Check sheet for the modelled part. Datum: model origin and axes. Units: mm. A direction names the side the tool comes from. Coordinates: 2 decimals unless noted, no trailing zeros. Loops run counter-clockwise (first coordinate to the right, second up) from the corner with the lowest first, then second, coordinate; pieces in that order, holes last. Notation, with made-up numbers: (13.25, -2.75) -> (17.25, -2.75) arc R20 cw to (17.25, 2.25) -> close; hole circle Ø3 at (9, 38). An arc over 180 degrees is marked (long way). Use one line per item in the form item = value.
from build123d import *

# Parameters (mm, degrees)
F1_DEPTH = 26
F2_SIZE  = 0.8


with BuildPart() as f1:
    # F0 (on Front) → F1 (new body)
    with BuildSketch(Plane.XZ):
        Polygon((-14.5, 0), (0, 0), (0, 2), (-13, 2), (-13, 12), (-10, 12), (-10, 13.5), (-14.5, 13.5), align=None)
    extrude(amount=-F1_DEPTH)

    # F2
    f2_edges = [f1.edges().sort_by_distance(p)[0] for p in [
        (-10, 13, 12),
    ]]
    chamfer(f2_edges, length=F2_SIZE)

    # F3: F1 across plane


with BuildPart() as f1_1:
    add(f1.part)
    add(f1.part.mirror(Plane.YZ))


solid = f1_1.part
(1) Scan lines: line 1 along X through (y, z) = (6, 13); line 2 along X through (y, z) = (12.5, 8.75); line 3 along Z through (x, y) = (-11.25, 14.5). Record each from-to range of solid material in increasing order.
Established:
line_1 = -14.5 to -10, 10 to 14.5
line_2 = -14.5 to -13, 13 to 14.5
line_3 = 0 to 2, 12 to 13.5
(2) Mould release check, pull along X, two halves, no side actions. Record for faces 3 (the flat face through (12, 13, 13.5)), 4 (the flat face through (-13, 13, 7)), 5 (the flat face through (14.5, 13, 7)): +X half, -X half, draft (parallel to the pull), parting line (faces both ways), or undercut.
Established:
face_3 = draft
face_4 = undercut
face_5 = +X half
(3) Section check C-C, the plane x = -12.5. Record the boundary of the cut face in (y, z), plus the area to 3 significant figures.
Established:
outline = (0, 0) -> (26, 0) -> (26, 2) -> (0, 2) -> close; (0, 12) -> (26, 12) -> (26, 13.5) -> (0, 13.5) -> close
area = 91.0 mm²
(4) Section check D-D, the plane x = 9. Record the boundary of the cut face in (y, z).
Established:
outline = (0, 0) -> (26, 0) -> (26, 2) -> (0, 2) -> close
(5) Tool access check on faces 1 (the flat face through (0, 13, 0)), 2 (the flat face through (-12, 13, 12)). Record the directions out of +Z, -Z, +X, -X, +Y, -Y that give a thin tool (end or side, any length) a straight path to the whole face; none if there is none.
Established:
face_1 = -Z, +X, -X, +Y, -Y
face_2 = +Y, -Y
(6) Section check B-B, the plane y = 7.5. Record the boundary of the cut face in (x, z).
Established:
outline = (-14.5, 0) -> (14.5, 0) -> (14.5, 13.5) -> (10, 13.5) -> (10, 12.8) -> (10.8, 12) -> (13, 12) -> (13, 2) -> (-13, 2) -> (-13, 12) -> (-10.8, 12) -> (-10, 12.8) -> (-10, 13.5) -> (-14.5, 13.5) -> close
(7) Section check A-A, the plane z = 6. Record the boundary of the cut face in (x, y), plus the area to 3 significant figures.
Established:
outline = (-14.5, 0) -> (-13, 0) -> (-13, 26) -> (-14.5, 26) -> close; (13, 0) -> (14.5, 0) -> (14.5, 26) -> (13, 26) -> close
area = 78.0 mm²
